from build123d import *

# Parameters (mm, degrees)
F2_R = 2


with BuildPart() as f1:
    # F0 (on Front) → F1 (revolve)
    with BuildSketch(Plane.XZ):
        with BuildLine():
            Line((-2.35, 0), (0, 0))
            Line((0, 0), (0, 7.84415))
            ThreePointArc((0, 7.84415), (-3.725421, 8.502268), (-7, 10.396736))
            Line((-7, 10.396736), (-8.5, 10.396736))
            Line((-8.5, 10.396736), (-8.5, 7.5))
            Line((-8.5, 7.5), (-2.35, 7.5))
            Line((-2.35, 7.5), (-2.35, 0))
        make_face()
    revolve(axis=Axis((0, 0, 3.922075), (0, 0, -1)))

    # F2
    f2_edges = [f1.edges().sort_by_distance(p)[0] for p in [
        (7, 0, 10.396736),
    ]]
    fillet(f2_edges, radius=F2_R)


solid = f1.part
Read the model definition and answer for the solid it produces. Units are mm, in the model's axes. A direction names the side the tool comes from. Give positions to 0.01 mm unless a question says otherwise; leave off trailing zeros. Loops run counter-clockwise (first coordinate to the right, second up) from the corner with the lowest first, then second, coordinate; pieces in that order, holes last. Notation, with made-up numbers: (8, 69.5) -> (66, 69.5) arc R36 ccw to (66, 104.5) -> close; hole circle Ø8 at (-17, 62.5). An arc over 180 degrees is marked (long way). Answer as CSV lines item,"result".
Item 1: Consider line 1 (Z direction, x = 3.25, y = 7.25); line 2 (Y direction, x = 7.75, z = 9); line 3 (Z direction, x = -3.5, y = 5.25). Determine where each line is inside the solid, lowest interval first. Write a range as [from, to].
Returned:
line 1,"z = [7.5, 10.4]"
line 2,"y = [-3.49, 3.49]"
line 3,"z = [7.5, 9.86]"
Item 2: Each of these flat-tipped pins is pushed along its axis until it touches: pin 1 (6 mm diameter, centred on y = 6.5, z = 6, fed in from +X); pin 2 (4 mm diameter, centred on x = -4.5, z = 7.5, fed in from +Y); pin 3 (3 mm diameter, centred on x = -4, y = -4, fed in from -Z). Where does it stop, or does it pass through?
Returned:
pin 1,"stops at x = 7.55"
pin 2,"stops at y = 8.12"
pin 3,"stops at z = 7.5"
Item 3: Find section A-A on z = 1. Give the vertices of the cut face in (x, y).
Returned:
outline,"circle Ø4.7 at (0, 0)"
Item 4: For faces 1 (the face through (0.509, -2.294, 3.698)), 2 (the face through (0, 0, 0)), determine the directions among +Z, -Z, +X, -X, +Y, -Y from which every point of the face is accessible in a straight line to the end or side of a thin tool.
Returned:
face 1,"-Z"
face 2,"-Z, +X, -X, +Y, -Y"
